Read the model definition and answer for the solid it produces. Units are mm, in the model's axes. A direction names the side the tool comes from. Give positions to 0.01 mm unless a question says otherwise; leave off trailing zeros. Loops run counter-clockwise (first coordinate to the right, second up) from the corner with the lowest first, then second, coordinate; pieces in that order, holes last. Notation, with made-up numbers: (52.25, 75) - (88.25, 75) arc R23 ccw to (88.25, 85) - close; hole circle Ø7 at (78, 11.25). An arc over 180 degrees is marked (long way). Write item = value, one per line.
```python
from build123d import *

# Parameters (mm, degrees)
BOSS_EXTRUDE2_DEPTH = 12.7
CIRPATTERN1_COUNT   = 18
CUT_EXTRUDE1_DEPTH  = 7.62
SKETCH5_W           = 2.032
SKETCH5_H           = 5.817262372
SKETCH6_R           = 1.905
CUT_EXTRUDE2_DEPTH  = 3.81
SKETCH7_R           = 1.905
BOSS_EXTRUDE3_DEPTH = 4.318
SKETCH8_R           = 4.40562407
CUT_EXTRUDE3_DEPTH  = 2.032


with BuildPart() as part:
    # Sketch2 → Boss-Extrude2 (new body)
    with BuildSketch(Plane.XY):
        with BuildLine():
            Line((-8.763, -27.305), (-2.184048035, -24.910457312))
            ThreePointArc((-2.184048035, -24.910457312), (-2.085861254, -25.19970624), (-2.000384787, -25.492962715))
            Line((-2.000384787, -25.492962715), (-0.773658987, -25.164262528))
            ThreePointArc((-0.773658987, -25.164262528), (-0.106264973, -25.122191283), (0.552010516, -25.239911886))
            ThreePointArc((0.552010516, -25.239911886), (0.633222569, -25.648192444), (0.696548377, -26.05962683))
            ThreePointArc((0.696548377, -26.05962683), (0.118234575, -26.395391489), (-0.523299868, -26.584119648))
            Line((-0.523299868, -26.584119648), (-1.788467135, -26.694807441))
            ThreePointArc((-1.788467135, -26.694807441), (-1.768489119, -26.99961306), (-1.761825553, -27.305))
            Line((-1.761825553, -27.305), (-8.763, -27.305))
        make_face()
    boss_extrude2 = extrude(amount=BOSS_EXTRUDE2_DEPTH)

    # CirPattern1: Boss-Extrude2 ×18 about axis
    cirpattern1_axis = Axis((-8.763, -27.305, 0), (0, 0, 1))
    for i in range(1, CIRPATTERN1_COUNT):
        add(boss_extrude2.rotate(cirpattern1_axis, i * 360 / CIRPATTERN1_COUNT))

    # Sketch4 → Cut-Extrude1 (cut)
    with BuildSketch(Plane(origin=(0, 0, 0), x_dir=(-1, 0, 0), z_dir=(0, 0, -1))):
        with BuildLine():
            Line((10.2489, -29.2862), (10.2489, -25.3238))
            ThreePointArc((10.2489, -25.3238), (8.763, -24.8285), (7.2771, -25.3238))
            Line((7.2771, -25.3238), (7.2771, -29.2862))
            ThreePointArc((7.2771, -29.2862), (8.763, -29.7815), (10.2489, -29.2862))
        make_face()
    extrude(amount=-CUT_EXTRUDE1_DEPTH, mode=Mode.SUBTRACT)

    # Sketch5 → Cut-Revolve1 (revolve, cut)
    with BuildSketch(Plane.ZY.offset(8.763), mode=Mode.PRIVATE) as cut_revolve1_sk:
        with Locations((1.016, -34.619255256)):
            Rectangle(SKETCH5_W, SKETCH5_H)
        with Locations((11.684, -34.619255256)):
            Rectangle(SKETCH5_W, SKETCH5_H)
    revolve(cut_revolve1_sk.sketch.rotate(Axis((-8.763, -27.305, 7.62), (0, 0, -1)), 270), axis=Axis((-8.763, -27.305, 7.62), (0, 0, -1)), mode=Mode.SUBTRACT)

    # Sketch6 → Cut-Extrude2 (cut)
    with BuildSketch(Plane.XY.offset(12.7)):
        with Locations((-8.763, -27.305)):
            Circle(SKETCH6_R)
    extrude(amount=-CUT_EXTRUDE2_DEPTH, mode=Mode.SUBTRACT)

    # Sketch7 → Boss-Extrude3 (add, symmetric)
    with BuildSketch(Plane(origin=(0, 0, 6.35), x_dir=(-1, 0, 0), z_dir=(0, 0, -1))):
        with BuildLine():
            Line((11.454508553, -23.650525812), (77.596423172, -39.896538245))
            ThreePointArc((77.596423172, -39.896538245), (80.666753219, -44.966255733), (75.597035731, -48.036585779))
            Line((75.597035731, -48.036585779), (9.455121112, -31.790573347))
            ThreePointArc((9.455121112, -31.790573347), (13.203025928, -28.395574968), (11.454508553, -23.650525812))
        make_face()
        with Locations((76.596729452, -43.966562012)):
            Circle(SKETCH7_R, mode=Mode.SUBTRACT)
    extrude(amount=BOSS_EXTRUDE3_DEPTH, both=True)

    # Sketch8 → Cut-Extrude3 (cut)
    with BuildSketch(Plane.XY.offset(10.668)):
        with Locations((-8.763, -27.305)):
            Circle(SKETCH8_R)
    extrude(amount=CUT_EXTRUDE3_DEPTH, mode=Mode.SUBTRACT)


solid = part.part
```
1) Each of these flat-tipped pins is pushed along its axis until it touches: P1, Ø1.1, axis at x = -8.5, y = -28, coming from the +Z side; P2, Ø2.5, axis at x = -76.6, y = -43.97, coming from the +Z side; P3, Ø5, axis at x = -27.5, z = 9, coming from the +Y side; P4, Ø2, axis at y = -31, z = 2, coming from the +X side. Where does it stop, or does it pass through?
Output:
P1 = 8.89
P2 = through
P3 = -26.98
P4 = -0.3
2) Find the intervals of material crossed by probe 1 along Y at (x, z) = (-7.5, 5.75); probe 2 along Y at (x, z) = (-75, 3.5); probe 3 along Z at (x, y) = (-51.5, -37), in increasing order.
Output:
probe_1 = -34.19 to -29.44, -25.17 to -20.42
probe_2 = -47.89 to -45.01, -42.93 to -39.26
probe_3 = 2.03 to 10.67
3) A tool of negligible diameter and unlimited length cuts with its end or side. For faces 5 (the face through (-47.425, -32.486, 6.29)), 6 (the face through (-0.097, -29.487, 6.29)), 7 (the face through (-8.74, -29.78, 3.76)), from which of +Z, -Z, +X, -X, +Y, -Y can it reach the whole face along a straight path? Write none if from no direction.
Output:
face_5 = +Z, -Z, -X, +Y
face_6 = +Z, -Z
face_7 = -Z
4) The mould has two halves that part along X. Classify faces 1 (the face through (-10.249, -27, 4)), 2 (the face through (-6.395, -31.02, 1.03)), 3 (the face through (-0.12, -25.12, 6.29)), 4 (the face through (-16.316, -24.845, 6.29)): pulls with the +X half, pulls with the -X half, needs draft (parallel to the pull), parting line crosses it, or undercut.
Output:
face_1 = undercut
face_2 = parting line crosses it
face_3 = undercut
face_4 = pulls with the -X half
5) A cutting plane is placed at B-B on y = -45. Determine the outline of the cut face in (x, z), then the cut area to 3 significant figures.
Output:
outline = (-80.66, 2.03) - (-78.2, 2.03) - (-78.2, 10.67) - (-80.66, 10.67) - close; (-75, 2.03) - (-63.23, 2.03) - (-63.23, 10.67) - (-75, 10.67) - close
area = 123 mm²
6) A cutting plane is placed at C-C on x = -27. Determine the outline of the cut face in (y, z), then the cut area to 3 significant figures.
Output:
outline = (-36.1, 2.03) - (-27.47, 2.03) - (-27.47, 10.67) - (-36.1, 10.67) - close
area = 74.5 mm²
7) A cutting plane is placed at A-A on z = 1. Determine the outline of the cut face in (x, y) (1 decimal).
Output:
outline = circle Ø8.8 at (-8.8, -27.3); hole (-10.2, -29.3) arc R2.5 ccw to (-7.3, -29.3) - (-7.3, -25.3) arc R2.5 ccw to (-10.2, -25.3) - close
